Can you work these out from the model? Positions are in its coordinate system, mm. Coordinates: 2 decimals unless noted, no trailing zeros. Order: outer loops, then holes, each group sorted by start corner. A loop starts at its lowest first (then second) coordinate and runs counter-clockwise, first axis right, second up. Notation, with made-up numbers: (-0.5, -5.5) -> (8.5, -5.5) arc R26 ccw to (8.5, 15.5) -> close; hole circle Ø10 at (48.25, -6.75). An arc over 180 degrees is marked (long way). Answer as CSV lines item,"result".
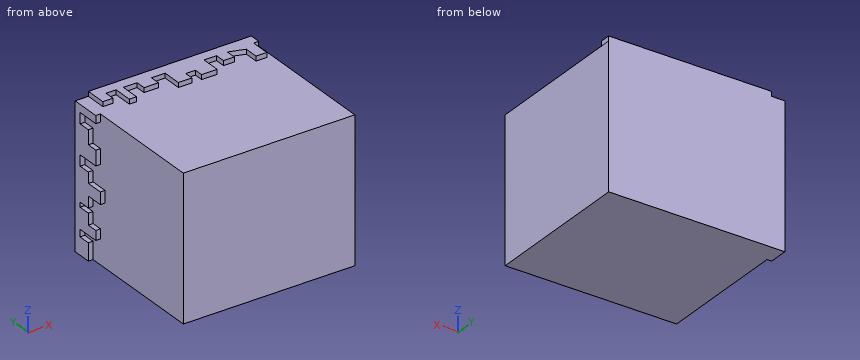
from build123d import *

# Parameters (mm, degrees)
F0_W     = 83.653443
F0_H     = 73.160328
F1_DEPTH = 69.596
F3_DEPTH = 2.286
F5_DEPTH = 2.286


with BuildPart() as f1:
    # F0 (on Top) → F1 (new body)
    with BuildSketch(Plane.XY):
        with Locations((-2.769016, 10.784589)):
            Rectangle(F0_W, F0_H)
    extrude(amount=F1_DEPTH)

    # F2 (on face) → F3 (join)
    with BuildSketch(Plane(origin=(-44.595737, 0, 0), x_dir=(0, -1, 0), z_dir=(-1, 0, 0))):
        Polygon((-47.364753, 0), (-38.037542, 0), (-38.037542, 8.452787), (-43.867048, 8.452787), (-43.867048, 11.950491), (-32.790981, 11.950491), (-32.790981, 16.6141), (-38.037542, 16.6141), (-38.037542, 22.152131), (-43.867048, 22.152131), (-43.867048, 24.483934), (-38.037542, 24.483934), (-38.037542, 30.021966), (-29.584754, 30.021966), (-29.584754, 35.851479), (-38.037542, 35.851479), (-38.037542, 41.098036), (-43.867048, 41.098036), (-43.867048, 46.344589), (-32.790981, 46.344589), (-32.790981, 53.631473), (-38.037542, 53.631473), (-38.037542, 60.626887), (-43.867048, 60.626887), (-43.867048, 65.873444), (-32.790981, 65.873444), (-32.790981, 69.596), (-47.364753, 69.596), align=None)
    extrude(amount=F3_DEPTH)

    # F4 (on face) → F5 (join)
    with BuildSketch(Plane.XY.offset(69.596)):
        Polygon((39.057706, 47.364753), (-40.410984, 47.364753), (-40.410984, 37.163116), (-35.455901, 37.163116), (-35.455901, 42.118195), (-30.50082, 42.118195), (-30.50082, 32.790981), (-27.003115, 32.790981), (-27.003115, 42.118195), (-20.299181, 42.118195), (-20.299181, 37.163116), (-13.303772, 37.163116), (-13.303772, 42.118195), (-6.599837, 42.118195), (-6.599837, 32.790981), (0, 32.790981), (0, 37.163116), (4.767703, 37.163116), (4.767703, 32.790981), (12.346066, 32.790981), (12.346066, 42.118195), (18.467048, 42.118195), (18.467048, 37.163116), (23.713607, 37.163116), (23.713607, 42.118195), (31.291965, 39.640656), (31.291965, 32.790981), (36.538523, 32.790981), (36.538523, 42.118195), (39.057706, 42.118195), align=None)
    extrude(amount=F5_DEPTH)


solid = f1.part
Q1. If I drill on line 1 (X direction, y = 25.5, z = 21); line 2 (Z direction, x = 21.5, y = -2), over which ranges is the centre line in solid material (lowest first)?
Solution:
line 1,"-44.6 to 39.06"
line 2,"0 to 69.6"
Q2. Imagine slicing it at B-B (x = -11.5). List the corners of the cut face in (y, z) for me, and give its area (3 significant figures).
Solution:
outline,"(-25.8, 0) -> (47.36, 0) -> (47.36, 71.88) -> (42.12, 71.88) -> (42.12, 69.6) -> (-25.8, 69.6) -> close"
area,"5,100 mm2"
Q3. Imagine slicing it at C-C (z = 64.5). List the corners of the cut face in (x, y) for me.
Solution:
outline,"(-46.88, 43.87) -> (-44.6, 43.87) -> (-44.6, -25.8) -> (39.06, -25.8) -> (39.06, 47.36) -> (-46.88, 47.36) -> close"
Q4. Imagine slicing it at A-A (y = 31). List the corners of the cut face in (x, z) for me, and give its area (3 significant figures).
Solution:
outline,"(-46.88, 30.02) -> (-44.6, 30.02) -> (-44.6, 0) -> (39.06, 0) -> (39.06, 69.6) -> (-44.6, 69.6) -> (-44.6, 35.85) -> (-46.88, 35.85) -> close"
area,"5,840 mm2"
Q5. Imagine slicing it at D-D (y = 4). List the corners of the cut face in (x, z) for me, and give its area (3 significant figures).
Solution:
outline,"(-44.6, 0) -> (39.06, 0) -> (39.06, 69.6) -> (-44.6, 69.6) -> close"
area,"5,820 mm2"
Q6. For P1, Ø0.7, axis at x = -46, z = 14.5, coming from the -Y side; P2, Ø1.1, axis at x = -46, y = 40.5, coming from the -Z side; P3, Ø2.5, axis at x = 17, z = 71, coming from the -Y side; P4, Ø5, axis at x = 4, y = 10.5, coming from the +Z side, each with a flat end and sliding along its axis, tell me the tip position at first contact or that it passes through.
Solution:
P1,"y = 32.79"
P2,"z = 0"
P3,"y = 42.12"
P4,"z = 69.6"
